Input: part model. Units: mm. Frame: model coordinates. Round coordinates to 2 decimals unless told otherwise and drop trailing zeros. Order: outer loops, then holes, each group sorted by start corner. A loop starts at its lowest first (then second) coordinate and runs counter-clockwise, first axis right, second up. Notation, with made-up numbers: (-10.5, 81) -> (-0.5, 81) arc R26 ccw to (-0.5, 110) -> close; hole circle Ø4 at (-33.75, 16). An arc over 180 degrees is marked (long way). Use a Markdown table: item, result.
from build123d import *

# Parameters (mm, degrees)
SKETCH1_W            = 132
SKETCH1_H            = 10
BOSS_EXTRUDE1_DEPTH  = 76.2
CUT_EXTRUDE1_DEPTH   = 76.2
FILLET2_R            = 2
M4_CLEARANCE_HOLE1_D = 4.5


with BuildPart() as part:
    # Sketch1 → Boss-Extrude1 (new body)
    with BuildSketch(Plane.XY):
        with Locations((0, 5)):
            Rectangle(SKETCH1_W, SKETCH1_H)
    extrude(amount=BOSS_EXTRUDE1_DEPTH)

    # Sketch2 → Cut-Extrude1 (cut)
    with BuildSketch(Plane.XY.offset(76.2)):
        Polygon((34.226497308, 0), (37.113248654, -5), (42.886751346, -5), (45.773502692, 0), (42.886751346, 5), (37.113248654, 5), align=None)
        Polygon((-37.113248654, 5), (-34.226497308, 0), (-37.113248654, -5), (-42.886751346, -5), (-45.773502692, 0), (-42.886751346, 5), align=None)
    extrude(amount=-CUT_EXTRUDE1_DEPTH, mode=Mode.SUBTRACT)

    # Fillet2
    fillet2_edges = [part.edges().sort_by_distance(p)[0] for p in [
        (66, 10, 38.1),
        (-66, 10, 38.1),
    ]]
    fillet(fillet2_edges, radius=FILLET2_R)

    # M4 Clearance Hole1 (through all)
    with Locations(Plane(origin=(0, 10, 0), x_dir=(1, 0, 0), z_dir=(0, 1, 0))):
        with Locations((-56, -67), (-56, -9), (56, -9), (56, -67)):
            Hole(M4_CLEARANCE_HOLE1_D / 2)


solid = part.part
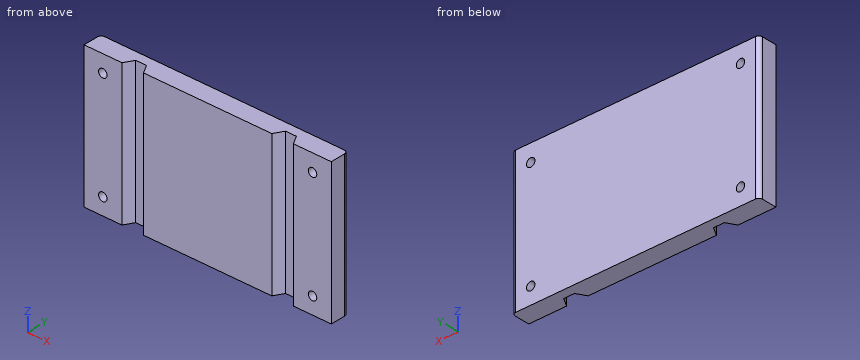
1) Cut plane A-A on y = 3. Return loops of the section in (x, z), and give its area (3 significant figures).
Results found:
| item | result |
|---|---|
| outline | (-66, 0) -> (-44.04, 0) -> (-44.04, 76.2) -> (-66, 76.2) -> close; (-35.96, 0) -> (35.96, 0) -> (35.96, 76.2) -> (-35.96, 76.2) -> close; (44.04, 0) -> (66, 0) -> (66, 76.2) -> (44.04, 76.2) -> close; hole circle Ø4.5 at (-56, 9); hole circle Ø4.5 at (-56, 67); hole circle Ø4.5 at (56, 9); hole circle Ø4.5 at (56, 67) |
| area | 8,760 mm² |
2) Line query: L1, parallel to X at y = 6.25, z = 9; L2, parallel to Z at x = -56, y = 7.75; L3, parallel to X at y = 2.75, z = 73.5. Output: solid intervals per line, ascending. Write a range as [from, to].
Results found:
| item | result |
|---|---|
| L1 | x = [-66, -58.25], [-53.75, 53.75], [58.25, 66] |
| L2 | z = [0, 6.75], [11.25, 64.75], [69.25, 76.2] |
| L3 | x = [-66, -44.19], [-35.81, 35.81], [44.19, 66] |
3) Cut plane D-D on z = 51. Return loops of the section in (x, y).
Results found:
| item | result |
|---|---|
| outline | (-66, 0) -> (-45.77, 0) -> (-42.89, 5) -> (-37.11, 5) -> (-34.23, 0) -> (34.23, 0) -> (37.11, 5) -> (42.89, 5) -> (45.77, 0) -> (66, 0) -> (66, 8) arc R2 ccw to (64, 10) -> (-64, 10) arc R2 ccw to (-66, 8) -> close |
4) Cut plane C-C on z = 9. Return loops of the section in (x, y), and give its area (3 significant figures).
Results found:
| item | result |
|---|---|
| outline | (-66, 0) -> (-58.25, 0) -> (-58.25, 10) -> (-64, 10) arc R2 ccw to (-66, 8) -> close; (-53.75, 0) -> (-45.77, 0) -> (-42.89, 5) -> (-37.11, 5) -> (-34.23, 0) -> (34.23, 0) -> (37.11, 5) -> (42.89, 5) -> (45.77, 0) -> (53.75, 0) -> (53.75, 10) -> (-53.75, 10) -> close; (58.25, 0) -> (66, 0) -> (66, 8) arc R2 ccw to (64, 10) -> (58.25, 10) -> close |
| area | 1,140 mm² |
5) Pin query (flat end, axial travel): pin 1 Ø1.7 at (x, z) = (39, 48.5) entering from -Y. Return the tip coordinate at first contact, or that it passes through.
Results found:
| item | result |
|---|---|
| pin 1 | stops at y = 5 |
6) Cut plane B-B on x = -56. Return loops of the section in (y, z), and give its area (3 significant figures).
Results found:
| item | result |
|---|---|
| outline | (0, 0) -> (10, 0) -> (10, 6.75) -> (0, 6.75) -> close; (0, 11.25) -> (10, 11.25) -> (10, 64.75) -> (0, 64.75) -> close; (0, 69.25) -> (10, 69.25) -> (10, 76.2) -> (0, 76.2) -> close |
| area | 672 mm² |
